```python
from build123d import *

# Parameters (mm, degrees)
F0_R          = 15.875
F0_R_2        = 6.35
F1_DEPTH      = 31.75
F2_DEPTH      = 31.75
F2_DEPTH_BACK = 44.45
F3_R          = 4.445
F4_DEPTH      = 76.2
F4_DEPTH_BACK = 76.2


with BuildPart() as f1:
    # F0 (on Top) → F1 (new body)
    with BuildSketch(Plane.XY):
        Circle(F0_R)
        Circle(F0_R_2, mode=Mode.SUBTRACT)
    extrude(amount=F1_DEPTH)

    # F0 (on Top) → F2 (join, two sides)
    with BuildSketch(Plane.XY) as f2_sk:
        Circle(F0_R_2)
    extrude(amount=F2_DEPTH)
    extrude(f2_sk.sketch, amount=-F2_DEPTH_BACK)

    # F3 (on Right) → F4 (join, two sides)
    with BuildSketch(Plane.YZ) as f4_sk:
        with Locations((0, 15.875)):
            Circle(F3_R)
    extrude(amount=F4_DEPTH)
    extrude(f4_sk.sketch, amount=-F4_DEPTH_BACK)

    # F5 (on face) → F6 (revolve)
    with BuildSketch(Plane.YZ.offset(76.2)):
        with BuildLine():
            Line((4.445, 15.875), (10.16, 15.875))
            ThreePointArc((10.16, 15.875), (0, 26.035), (-10.16, 15.875))
            Line((-10.16, 15.875), (-4.445, 15.875))
            ThreePointArc((-4.445, 15.875), (0, 20.32), (4.445, 15.875))
        make_face()
        with BuildLine():
            Line((-4.445, 15.875), (4.445, 15.875))
            ThreePointArc((4.445, 15.875), (0, 20.32), (-4.445, 15.875))
        make_face()
        with BuildLine():
            ThreePointArc((-4.445, 15.875), (0, 11.43), (4.445, 15.875))
            Line((4.445, 15.875), (-4.445, 15.875))
        make_face()
    revolve(axis=Axis((76.2, 0, 15.875), (0, 1, 0)))

    # F7 (on face) → F8 (revolve)
    with BuildSketch(Plane(origin=(-76.2, 0, 0), x_dir=(0, -1, 0), z_dir=(-1, 0, 0))):
        with BuildLine():
            Line((4.445, 15.875), (10.16, 15.875))
            ThreePointArc((10.16, 15.875), (0, 26.035), (-10.16, 15.875))
            Line((-10.16, 15.875), (-4.445, 15.875))
            ThreePointArc((-4.445, 15.875), (0, 20.32), (4.445, 15.875))
        make_face()
        with BuildLine():
            Line((-4.445, 15.875), (4.445, 15.875))
            ThreePointArc((4.445, 15.875), (0, 20.32), (-4.445, 15.875))
        make_face()
        with BuildLine():
            ThreePointArc((-4.445, 15.875), (0, 11.43), (4.445, 15.875))
            Line((4.445, 15.875), (-4.445, 15.875))
        make_face()
    revolve(axis=Axis((-76.2, 0, 15.875), (0, -1, 0)))


solid = f1.part
```
CAD build for the part. Positions are in the model's coordinates, mm. A direction names the side the tool comes from. Round coordinates to 2 decimals unless told otherwise and drop trailing zeros. Loops run counter-clockwise (first coordinate to the right, second up) from the corner with the lowest first, then second, coordinate; pieces in that order, holes last. Notation, with made-up numbers: (1, -37) - (58, -37) arc R15 cw to (58, -19) - close; hole circle Ø3 at (6, 82.5). An arc over 180 degrees is marked (long way). Return JSON: item names as keys, results as strings. Group by question number.
Q1. Band-saw the part on B-B on x = 0. Give the cut face in (y, z) (3 decimals).
Q2. Band-saw the part on A-A on y = 0. Give the cut face in (x, z) (3 decimals), plus the area to 3 significant figures.
Q3. Flat gauge pins, fed straight in: pin 1 Ø6 at (x, y) = (48, 2) entering from -Z; pin 2 Ø4.5 at (y, z) = (-1.5, 17.5) entering from +X; pin 3 Ø12 at (y, z) = (-1, -35) entering from +X; pin 4 Ø12 at (x, z) = (25.5, 0.5) entering from -Y. Where does each tip first touch, or does it go through?
Q4. Tool access for faces 5 (the face through (7, 0, 0)), 6 (the face through (0, 0, 31.75)), 7 (the face through (-40.79, -0.58, 20.28)): list every direction of +Z, -Z, +X, -X, +Y, -Y with a clear straight run to the whole face (end or side of a thin tool).
Q5. Drill centre lines: line 1 along X through (y, z) = (4.5, 15.5); line 2 along X through (y, z) = (0.5, 18); line 3 along X through (y, z) = (0.5, -15.5). Where is each one in solid material? Low to high. Write a range as [from, to].
Q6. Band-saw the part on D-D on x = 58. Give the cut face in (y, z) (3 decimals), plus the area to 3 significant figures.
Q7. Band-saw the part on C-C on z = -36.5. Give the cut face in (x, y), plus the area to 3 significant figures.
Q8. Two-plate mould, pull along Y, no slides. Class faces 1 (the face through (-76.2, 0, 16)), 2 (the face through (40.79, -0.58, 20.28)), 3 (the face through (0, 0, -44.45)), 4 (the face through (76.2, 0, 16)): +Y half, -Y half, draft (parallel to the pull), parting line (faces both ways), or undercut.
Solutions:
{
 "1": {"outline": "(-15.875, 0) - (-6.35, 0) - (-6.35, -44.45) - (6.35, -44.45) - (6.35, 0) - (15.875, 0) - (15.875, 31.75) - (-15.875, 31.75) - close"},
 "2": {"outline": "(-67.064, 11.43) - (-15.875, 11.43) - (-15.875, 0) - (-6.35, 0) - (-6.35, -44.45) - (6.35, -44.45) - (6.35, 0) - (15.875, 0) - (15.875, 11.43) - (67.064, 11.43) arc R10.16 ccw (long way) to (67.064, 20.32) - (15.875, 20.32) - (15.875, 31.75) - (-15.875, 31.75) - (-15.875, 20.32) - (-67.064, 20.32) arc R10.16 ccw (long way) to start; hole (-76.2, 11.43) - (-76.2, 20.32) arc R4.445 ccw to start; hole (76.2, 11.43) arc R4.445 ccw to (76.2, 20.32) - close", "area": "3,060 mm^2"},
 "3": {"pin 1": "stops at z = 11.43", "pin 2": "stops at x = 86.36", "pin 3": "stops at x = 6.35", "pin 4": "passes through"},
 "4": {"face 5": "-Z", "face 6": "+Z, +X, -X, +Y, -Y", "face 7": "none"},
 "5": {"line 1": "x = [-85.3, -67.1], [-15.22, 15.22], [67.1, 85.3]", "line 2": "x = [-86.12, -80.07], [-76.2, 76.2], [80.07, 86.12]", "line 3": "x = [-6.33, 6.33]"},
 "6": {"outline": "circle Ø8.89 at (0, 15.875)", "area": "62.1 mm^2"},
 "7": {"outline": "circle Ø12.7 at (0, 0)", "area": "127 mm^2"},
 "8": {"face 1": "undercut", "face 2": "parting line", "face 3": "draft", "face 4": "undercut"}
}
